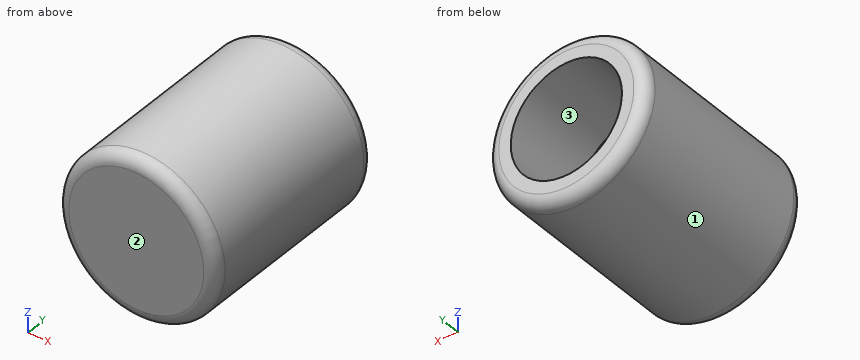
from build123d import *

# Parameters (mm, degrees)
SKETCH_1_R               = 11
SKETCH_1_R_2             = 8.1
EXTRUDE_1_DEPTH          = 11
SWEEP_2_PITCH            = 2
CUT_EXTRUDE_1_DEPTH      = 20.256876011
CUT_EXTRUDE_1_DEPTH_BACK = 20.256876011
SKETCH_8_W               = 20.965644498
SKETCH_8_H               = 3.347195004
CUT_EXTRUDE_2_DEPTH      = 1
SKETCH_1_3_R             = 20
SKETCH_1_3_R_2           = 14
EXTRUDE_2_DEPTH          = 31
SKETCH_2_R               = 20
EXTRUDE_4_DEPTH          = 20
FILLET_1_R               = 3


with BuildPart() as part:
    # Sketch 1 → Extrude 1 (new body)
    with BuildSketch(Plane(origin=(0, 0, 0), x_dir=(1, 0, 0), z_dir=(0, 1, 0))):
        with Locations(Location((0, 0, 0), (0, 0, 270))):
            Circle(SKETCH_1_R)
        with Locations(Location((0, 0, 0), (0, 0, 270))):
            Circle(SKETCH_1_R_2, mode=Mode.SUBTRACT)
    extrude(amount=EXTRUDE_1_DEPTH)

    # Sweep 2: the profile of Sketch 7 profile screwed along a right-hand helix of 5.5 turns, 10 arcs to a turn; built about Z, then put on its axis
    sweep_2_z = Axis((0, 0, 0), (0, 0, 1))
    sweep_2_corners = [(8.1003, 0, 0.35021), (8.1003, 0, -0.35021), (7.6, 0, 0)]
    with BuildLine(mode=Mode.PRIVATE) as sweep_2_profile:
        Line(sweep_2_corners[0], sweep_2_corners[1])
        Line(sweep_2_corners[1], sweep_2_corners[2])
        Line(sweep_2_corners[2], sweep_2_corners[0])
    sweep_2_cap = Face(sweep_2_profile.wire())
    sweep_2_turn_angles = [0, 18, 36, 54, 72, 90, 108, 126, 144, 162, 180, 198, 216, 234, 252, 270, 288, 306, 324, 342, 360]
    sweep_2_turn_weights = [1, 0.9510565162951535, 1, 0.9510565162951535, 1, 0.9510565162951535, 1, 0.9510565162951535, 1, 0.9510565162951535, 1, 0.9510565162951535, 1, 0.9510565162951535, 1, 0.9510565162951535, 1, 0.9510565162951535, 1, 0.9510565162951535, 1]
    sweep_2_turn_rails = [Edge.make_bspline([Vector(p[0], p[1], 0).rotate(sweep_2_z, sweep_2_turn_angles[k]) / sweep_2_turn_weights[k] + Vector(0, 0, p[2] + SWEEP_2_PITCH * sweep_2_turn_angles[k] / 360) for k in range(21)], [0, 0, 0, 1, 1, 2, 2, 3, 3, 4, 4, 5, 5, 6, 6, 7, 7, 8, 8, 9, 9, 10, 10, 10], 2, sweep_2_turn_weights) for p in sweep_2_corners]
    sweep_2_turn_sides = [Face.make_surface_from_curves(sweep_2_turn_rails[p[0]], sweep_2_turn_rails[p[1]]) for p in [(0, 1), (1, 2), (2, 0)]]
    sweep_2_last_angles = [1800, 1818, 1836, 1854, 1872, 1890, 1908, 1926, 1944, 1962, 1980]
    sweep_2_last_weights = [1, 0.9510565162951535, 1, 0.9510565162951535, 1, 0.9510565162951535, 1, 0.9510565162951535, 1, 0.9510565162951394, 1]
    sweep_2_last_rails = [Edge.make_bspline([Vector(p[0], p[1], 0).rotate(sweep_2_z, sweep_2_last_angles[k]) / sweep_2_last_weights[k] + Vector(0, 0, p[2] + SWEEP_2_PITCH * sweep_2_last_angles[k] / 360) for k in range(11)], [0, 0, 0, 1, 1, 2, 2, 3, 3, 4, 4, 5, 5, 5], 2, sweep_2_last_weights) for p in sweep_2_corners]
    sweep_2_last_sides = [Face.make_surface_from_curves(sweep_2_last_rails[p[0]], sweep_2_last_rails[p[1]]) for p in [(0, 1), (1, 2), (2, 0)]]
    sweep_2 = Plane(origin=(0, 11, 0), x_dir=(-0.7071067811865537, 0, -0.7071067811865414), z_dir=(0, -1, 0)) * Solid(Shell([*[p.moved(Location((0, 0, SWEEP_2_PITCH * i))) for i in range(5) for p in sweep_2_turn_sides], *sweep_2_last_sides, sweep_2_cap, sweep_2_cap.rotate(sweep_2_z, 1980).moved(Location((0, 0, SWEEP_2_PITCH * 1980 / 360)))]))
    add(sweep_2)

    # Sketch 8 → Cut-Extrude 1 (cut, two sides: drawn at the far end of the back side and taken through both)
    with BuildSketch(Plane(origin=(0, 0, 0), x_dir=(-0.7071067811865536, 0, -0.7071067811865416), z_dir=(0.7071067811865416, 0, -0.7071067811865536)).offset(-CUT_EXTRUDE_1_DEPTH_BACK)):
        with Locations((0.517177751, 12.673597502)):
            Rectangle(SKETCH_8_W, SKETCH_8_H)
    extrude(amount=CUT_EXTRUDE_1_DEPTH + CUT_EXTRUDE_1_DEPTH_BACK, mode=Mode.SUBTRACT)

    # Sketch 9 → Cut-Extrude 2 (cut)
    with BuildSketch(Plane(origin=(0, 11, 0), x_dir=(1, 0, 0), z_dir=(0, 1, 0))):
        Polygon((-5.727564928, 5.727564928), (-4.090744655, 6.349136352), (-5.001356228, 5.001356228), align=None)
    extrude(amount=-CUT_EXTRUDE_2_DEPTH, mode=Mode.SUBTRACT)



with BuildPart() as body_2:
    # Sketch 1_3 → Extrude 2 (new body)
    with BuildSketch(Plane(origin=(0, 0, 0), x_dir=(1, 0, 0), z_dir=(0, 1, 0))):
        with Locations(Location((0, 0, 0), (0, 0, 270))):
            Circle(SKETCH_1_3_R)
        with Locations(Location((0, 0, 0), (0, 0, 270))):
            Circle(SKETCH_1_3_R_2, mode=Mode.SUBTRACT)
    extrude(amount=EXTRUDE_2_DEPTH)


with BuildPart() as part_1:
    add(part.part)

    add(body_2.part)  # Extrude 4 merges body 2
    # Sketch 2 → Extrude 4 (add)
    with BuildSketch(Plane.XZ):
        with Locations(Location((0, 0, 0), (0, 0, 270))):
            Circle(SKETCH_2_R)
    extrude(amount=EXTRUDE_4_DEPTH)

    # Fillet 1
    # the kernel refuses this fillet: 3 mm, written as the material it takes off along each edge
    with BuildSketch(Plane(origin=(0, 31, 0), x_dir=(0, 0, 1), z_dir=(-1, 0, 0))) as fillet_1_piece_1:
        with BuildLine():
            CenterArc((20 - FILLET_1_R, -FILLET_1_R), FILLET_1_R, 0, 90)
            Line((20, -FILLET_1_R), (20, 0))
            Line((20, 0), (20 - FILLET_1_R, 0))
        make_face()
    revolve(axis=Axis((0, 31, 0), (0, 1, 0)), mode=Mode.SUBTRACT)
    with BuildSketch(Plane(origin=(0, -20, 0), x_dir=(0, 0, -1), z_dir=(-1, 0, 0))) as fillet_1_piece_2:
        with BuildLine():
            CenterArc((20 - FILLET_1_R, -FILLET_1_R), FILLET_1_R, 0, 90)
            Line((20 - FILLET_1_R, 0), (20, 0))
            Line((20, 0), (20, -FILLET_1_R))
        make_face()
    revolve(axis=Axis((0, -20, 0), (0, -1, 0)), mode=Mode.SUBTRACT)


solid = part_1.part
Design review of the part built by this model. Coordinates are the model's own, in mm. Face numbers are marked on the shaded views. Round coordinates to 2 decimals unless told otherwise and drop trailing zeros. Order: outer loops, then holes, each group sorted by start corner. A loop starts at its lowest first (then second) coordinate and runs counter-clockwise, first axis right, second up.
1) Consider section B-B (y = -16). State the section outline as (x, z) points.
The answers:
outline: circle Ø40 at (0, 0)
2) Clearance check with flat-ended pins moving along their axes: pin 1 Ø8.5 at (x, z) = (-6, -4) entering from +Y; pin 2 Ø12 at (x, y) = (8, 19.5) entering from -Z; pin 3 Ø10 at (x, y) = (-11.5, 5.5) entering from +Z; pin 4 Ø24 at (x, z) = (-5, -4) entering from +Y. State where each tip first meets the part, or that it passes through.
The answers:
pin 1: stops at y = 11
pin 2: stops at z = -19.9
pin 3: stops at z = 18.91
pin 4: stops at y = 31
3) For L1, parallel to X at y = 0.75, z = 0; L2, parallel to X at y = 8, z = 0; L3, parallel to Z at x = -0.5, y = 24.5, list the stretches that pass through material, from the lowest coordinate up.
The answers:
L1: x = -20 to -14, -11 to -8.1, 8.1 to 11, 14 to 20
L2: x = -20 to -14, -11 to -8.1, 7.96 to 11, 14 to 20
L3: z = -19.99 to -13.99, 13.99 to 19.99
4) Consider section A-A (y = 20). State the section outline as (x, z) points, plus the area to 3 significant figures.
The answers:
outline: circle Ø40 at (0, 0); hole circle Ø28 at (0, 0)
area: 641 mm2
5) Draft analysis for pull direction X (two halves, no side actions). For the marked faces 1, 2 and 3, state which applies: released by +X, released by -X, zero draft, split by the parting line, or undercut.
The answers:
face 1: split by the parting line
face 2: zero draft
face 3: undercut
